Can you work these out from the model? Positions are in its coordinate system, mm. Face numbers are marked on the shaded views. A direction names the side the tool comes from. Give positions to 0.01 mm unless a question says otherwise; leave off trailing zeros. Loops run counter-clockwise (first coordinate to the right, second up) from the corner with the lowest first, then second, coordinate; pieces in that order, holes last. Notation, with made-up numbers: (11, 4.25) - (58, 4.25) arc R23 cw to (58, 22.25) - close; hole circle Ø6 at (-35.75, 58.5). An arc over 180 degrees is marked (long way). Answer in a Markdown table with one row per item.
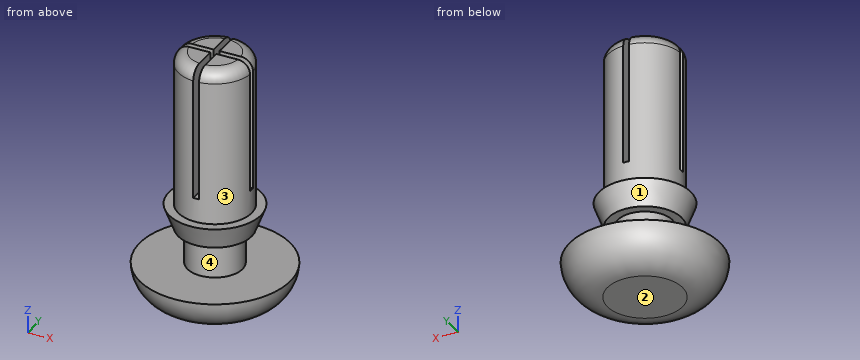
from build123d import *

# Parameters (mm, degrees)
SKETCH3_W          = 0.247904
SKETCH3_H          = 0.247904
CUT_EXTRUDE1_DEPTH = 5.588
FILLET1_R          = 0.508


with BuildPart() as part:
    # Sketch2 → Revolve1 (revolve)
    with BuildSketch(Plane(origin=(0, 0, 0), x_dir=(0, 0, -1), z_dir=(1, 0, 0))):
        with BuildLine():
            Line((2.54, 3.175), (2.54, 1.16205))
            Line((2.54, 1.16205), (1.016, 1.16205))
            Line((1.016, 1.16205), (1.016, 1.5494))
            Line((1.016, 1.5494), (0, 1.93675))
            Line((0, 1.93675), (0, 1.5494))
            Line((0, 1.5494), (-6.604, 1.5494))
            Line((-6.604, 1.5494), (-6.604, 0))
            Line((-6.604, 0), (4.064, 0))
            Line((4.064, 0), (4.064, 1.5875))
            ThreePointArc((4.064, 1.5875), (3.621333791, 2.687810439), (2.54, 3.175))
        make_face()
    revolve(axis=Axis((0, 0, 6.604), (0, 0, -1)))

    # Sketch3 → Cut-Extrude1 (cut)
    with BuildSketch(Plane.XY.offset(6.604)):
        with BuildLine():
            Line((0.123952, 3.172579534), (-0.123952, 3.172579534))
            Line((-0.123952, 3.172579534), (-0.123952, 1.544433962))
            ThreePointArc((-0.123952, 1.544433962), (0, 1.5494), (0.123952, 1.544433962))
            Line((0.123952, 1.544433962), (0.123952, 3.172579534))
        make_face()
        with BuildLine():
            ThreePointArc((0.123952, 1.544433962), (0, 1.5494), (-0.123952, 1.544433962))
            Line((-0.123952, 1.544433962), (-0.123952, 0.123952))
            Line((-0.123952, 0.123952), (0.123952, 0.123952))
            Line((0.123952, 0.123952), (0.123952, 1.544433962))
        make_face()
        with BuildLine():
            ThreePointArc((-1.544433962, -0.123952), (-1.5494, 0), (-1.544433962, 0.123952))
            Line((-1.544433962, 0.123952), (-3.172579534, 0.123952))
            Line((-3.172579534, 0.123952), (-3.172579534, -0.123952))
            Line((-3.172579534, -0.123952), (-1.544433962, -0.123952))
        make_face()
        with BuildLine():
            Line((3.172579534, 0.123952), (1.544433962, 0.123952))
            ThreePointArc((1.544433962, 0.123952), (1.548157993, 0.06202572), (1.5494, 0))
            ThreePointArc((1.5494, 0), (1.548157993, -0.06202572), (1.544433962, -0.123952))
            Line((1.544433962, -0.123952), (3.172579534, -0.123952))
            Line((3.172579534, -0.123952), (3.172579534, 0.123952))
        make_face()
        with BuildLine():
            Line((0.123952, -0.123952), (-0.123952, -0.123952))
            Line((-0.123952, -0.123952), (-0.123952, -1.544433962))
            ThreePointArc((-0.123952, -1.544433962), (0, -1.5494), (0.123952, -1.544433962))
            Line((0.123952, -1.544433962), (0.123952, -0.123952))
        make_face()
        with BuildLine():
            Line((1.544433962, 0.123952), (0.123952, 0.123952))
            Line((0.123952, 0.123952), (0.123952, -0.123952))
            Line((0.123952, -0.123952), (1.544433962, -0.123952))
            ThreePointArc((1.544433962, -0.123952), (1.548157993, -0.06202572), (1.5494, 0))
            ThreePointArc((1.5494, 0), (1.548157993, 0.06202572), (1.544433962, 0.123952))
        make_face()
        with BuildLine():
            Line((-0.123952, -0.123952), (-0.123952, 0.123952))
            Line((-0.123952, 0.123952), (-1.544433962, 0.123952))
            ThreePointArc((-1.544433962, 0.123952), (-1.5494, 0), (-1.544433962, -0.123952))
            Line((-1.544433962, -0.123952), (-0.123952, -0.123952))
        make_face()
        Rectangle(SKETCH3_W, SKETCH3_H)
        with BuildLine():
            ThreePointArc((0.123952, -1.544433962), (0, -1.5494), (-0.123952, -1.544433962))
            Line((-0.123952, -1.544433962), (-0.123952, -3.172579534))
            Line((-0.123952, -3.172579534), (0.123952, -3.172579534))
            Line((0.123952, -3.172579534), (0.123952, -1.544433962))
        make_face()
    extrude(amount=-CUT_EXTRUDE1_DEPTH, mode=Mode.SUBTRACT)

    # Fillet1
    fillet1_edges = [part.edges().sort_by_distance(p)[0] for p in [
        (1.095591247, -1.095591247, 6.604),
        (1.095591247, 1.095591247, 6.604),
        (-1.095591247, 1.095591247, 6.604),
        (-1.095591247, -1.095591247, 6.604),
    ]]
    fillet(fillet1_edges, radius=FILLET1_R)


solid = part.part
Q1. For pin 1 (1.5 mm diameter, centred on x = -0.5, z = 5, fed in from -Y); pin 2 (1.5 mm diameter, centred on y = 0, z = 2.5, fed in from +X); pin 3 (1.6 mm diameter, centred on x = -1, z = 4.5, fed in from +Y), each with a flat end and sliding along its axis, tell me the tip position at first contact or that it passes through.
Checked values:
| item | result |
|---|---|
| pin 1 | stops at y = -1.54 |
| pin 2 | stops at x = 1.54 |
| pin 3 | stops at y = 1.54 |
Q2. On a 3-axis mill with a long thin cutter (end or side, diameter ignored), from which of +Z, -Z, +X, -X, +Y, -Y can I reach the whole of each face in a straight line? I mean the marked faces 3 and 4. Say none if no direction works.
Checked values:
| item | result |
|---|---|
| face 3 | +Z |
| face 4 | none |
Q3. If we mould it in two halves opening along Z, with no side actions, what happens to the marked faces 1 and 2? For each: released by +Z, released by -Z, zero draft, split by the parting line, or undercut.
Checked values:
| item | result |
|---|---|
| face 1 | undercut |
| face 2 | released by -Z |
Q4. If I drill on line 1 (Y direction, x = -0.75, z = 2.25); line 2 (Y direction, x = -1, z = 2), over which ranges is the centre line in solid material (lowest first)? Write a range as [from, to].
Checked values:
| item | result |
|---|---|
| line 1 | y = [-1.36, -0.12], [0.12, 1.36] |
| line 2 | y = [-1.18, -0.12], [0.12, 1.18] |
Q5. Imagine slicing it at A-A, the plane z = 1.25. Write out the boundary of the cut face in (x, y).
Checked values:
| item | result |
|---|---|
| outline | (-1.54, -0.12) arc R1.55 ccw to (-0.12, -1.54) - (-0.12, -0.12) - close; (-1.54, 0.12) - (-0.12, 0.12) - (-0.12, 1.54) arc R1.55 ccw to start; (0.12, -1.54) arc R1.55 ccw to (1.54, -0.12) - (0.12, -0.12) - close; (0.12, 0.12) - (1.54, 0.12) arc R1.55 ccw to (0.12, 1.54) - close |
